The model under review builds one solid part; all positions refer to its coordinate system, in mm. Face numbers are marked on the shaded views. A direction names the side the tool comes from. Round coordinates to 2 decimals unless told otherwise and drop trailing zeros. Order: outer loops, then holes, each group sorted by start corner. A loop starts at its lowest first (then second) coordinate and runs counter-clockwise, first axis right, second up. Notation, with made-up numbers: (55.5, -28) - (111.5, -28) arc R14 cw to (111.5, -1) - close; hole circle Ø9 at (53.5, -29.5). An arc over 180 degrees is marked (long way). One line per question, with ' | ' between items. Start each with the question number.
Item 1: Insertion check: pin 1 Ø1 at (y, z) = (-0.5, 3.5) entering from -X; pin 2 Ø1 at (x, z) = (-0.5, 3) entering from +Y; pin 3 Ø1.6 at (y, z) = (0, 2.5) entering from +X. Each pin has a flat end and moves straight along its axis. Give the tip position at first contact, or say it passes through.
Item 2: Add section D-D on x = 3. State the section outline as (y, z) points.
Item 3: Add section C-C on z = 2.15. State the section outline as (x, y) points, and give its area (3 significant figures).
Item 4: Tool access review of the marked faces 1, 2, 3 and 4: name each direction out of +Z, -Z, +X, -X, +Y, -Y from which nothing blocks a thin tool from reaching the whole face with its end or side.
Item 5: Add section A-A on x = 1. State the section outline as (y, z) points.
Item 6: For L1, parallel to Y at x = 1.75, z = 1.5; L2, parallel to X at y = -1, z = 3.1; L3, parallel to Z at x = 3, y = 0.5, list the stretches that pass through material, from the lowest coordinate up. Write a range as [from, to].
Item 7: Add section B-B on y = -1.1. State the section outline as (x, z) points, and give its area (3 significant figures).
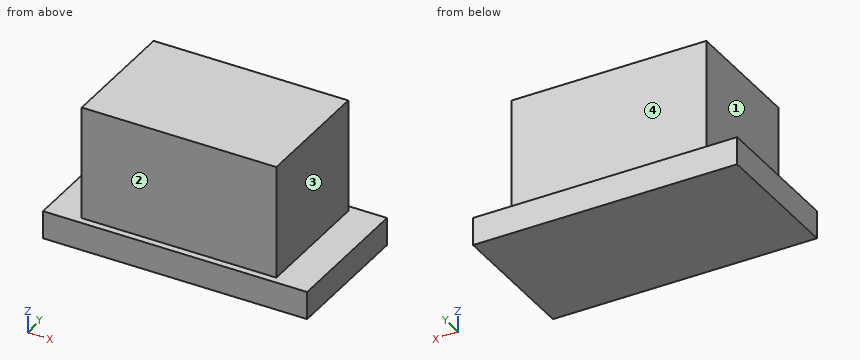
from build123d import *

# Parameters (mm, degrees)
SKETCH_1_W   = 7.6
SKETCH_1_H   = 4
FLANGE_DEPTH = 0.8
SKETCH_2_W   = 5.6
SKETCH_2_H   = 3.6
HEAD_DEPTH   = 4.06


with BuildPart() as part:
    # 草圖1 → flange (new body)
    with BuildSketch(Plane.XY):
        Rectangle(SKETCH_1_W, SKETCH_1_H)
    extrude(amount=FLANGE_DEPTH)

    # 草圖2 → head (add)
    with BuildSketch(Plane.XY):
        Rectangle(SKETCH_2_W, SKETCH_2_H)
    extrude(amount=HEAD_DEPTH)


solid = part.part
Determined:
1) pin 1: x = -2.8 | pin 2: y = 1.8 | pin 3: x = 2.8
2) outline: (-2, 0) - (2, 0) - (2, 0.8) - (-2, 0.8) - close
3) outline: (-2.8, -1.8) - (2.8, -1.8) - (2.8, 1.8) - (-2.8, 1.8) - close | area: 20.2 mm2
4) face 1: +Z, -X, +Y, -Y | face 2: +Z, +X, -X, -Y | face 3: +Z, +X, +Y, -Y | face 4: +Z, +X, -X, +Y
5) outline: (-2, 0) - (2, 0) - (2, 0.8) - (1.8, 0.8) - (1.8, 4.06) - (-1.8, 4.06) - (-1.8, 0.8) - (-2, 0.8) - close
6) L1: [-1.8, 1.8] | L2: [-2.8, 2.8] | L3: [0, 0.8]
7) outline: (-3.8, 0) - (3.8, 0) - (3.8, 0.8) - (2.8, 0.8) - (2.8, 4.06) - (-2.8, 4.06) - (-2.8, 0.8) - (-3.8, 0.8) - close | area: 24.3 mm2
